Geometry: final body of the model. Coordinates: model frame, mm. A direction names the side the tool comes from. Give positions to 0.01 mm unless a question says otherwise; leave off trailing zeros. Loops run counter-clockwise (first coordinate to the right, second up) from the corner with the lowest first, then second, coordinate; pieces in that order, holes last.
1. Section A-A, the plane z = 0. Output: boundary loops of the cut face in (x, y) (3 decimals).
2. Material intervals for line 1 along X through (y, z) = (1.5, -0.75); line 2 along X through (y, z) = (8, 0.75); line 3 along Z through (x, y) = (3.5, -1.5), sorted ascending.
3. First-contact query: P1, Ø1.5, axis at x = 11, y = -4.5, coming from the -Z side; P2, Ø8, axis at y = 2.5, z = 6, coming from the +X side; P3, Ø3, axis at x = 7, y = -8.5, coming from the -Z side. Flat tips, straight axial feed; report the tip coordinate or a pass-through.
4. Access query for faces 1 (the face through (36.7, 0, 0)), 2 (the face through (21, -2, 8)). Directions: +Z, -Z, +X, -X, +Y, -Y. A direction counts if a zero-diameter tool reaches every point of the face in a straight line with its end or side. Return the directions, or none.
5. Section C-C, the plane x = 32. Output: boundary loops of the cut face in (y, z), then the cut area to 3 significant figures.
6. Section D-D, the plane z = 7.25. Output: boundary loops of the cut face in (x, y), then the cut area to 3 significant figures.
from build123d import *

# Parameters (mm, degrees)
SKETCH_R     = 10.375
PAD_DEPTH    = 21
SKETCH001_R  = 7.875
PAD001_DEPTH = 4
SKETCH002_R  = 3
PAD002_DEPTH = 1.7
SKETCH003_R  = 1
PAD003_DEPTH = 10


with BuildPart() as part:
    # Sketch → Pad (new body)
    with BuildSketch(Plane.YZ):
        Circle(SKETCH_R)
    extrude(amount=PAD_DEPTH)

    # Sketch001 (on Face3 of Pad) → Pad001 (join)
    with BuildSketch(Plane.YZ.offset(21)):
        Circle(SKETCH001_R)
    extrude(amount=PAD001_DEPTH)

    # Sketch002 (on Face5 of Pad001) → Pad002 (join)
    with BuildSketch(Plane.YZ.offset(25)):
        Circle(SKETCH002_R)
    extrude(amount=PAD002_DEPTH)

    # Sketch003 (on Face7 of Pad002) → Pad003 (join)
    with BuildSketch(Plane.YZ.offset(26.7)):
        Circle(SKETCH003_R)
    extrude(amount=PAD003_DEPTH)


solid = part.part
Answers below:
1. outline: (0, -10.375) - (21, -10.375) - (21, -7.875) - (25, -7.875) - (25, -3) - (26.7, -3) - (26.7, -1) - (36.7, -1) - (36.7, 1) - (26.7, 1) - (26.7, 3) - (25, 3) - (25, 7.875) - (21, 7.875) - (21, 10.375) - (0, 10.375) - close
2. line 1: x = 0 to 26.7
2. line 2: x = 0 to 21
2. line 3: z = -10.27 to 10.27
3. P1: stops at z = -9.67
3. P2: stops at x = 26.7
3. P3: stops at z = -7.66
4. face 1: +Z, -Z, +X, +Y, -Y
4. face 2: +X
5. outline: circle Ø2 at (0, 0)
5. area: 3.14 mm2
6. outline: (0, -7.42) - (21, -7.42) - (21, -3.07) - (25, -3.07) - (25, 3.07) - (21, 3.07) - (21, 7.42) - (0, 7.42) - close
6. area: 336 mm2
